Build history of the part. All positions in model axes, mm. A direction names the side the tool comes from. Round coordinates to 2 decimals unless told otherwise and drop trailing zeros. Order: outer loops, then holes, each group sorted by start corner. A loop starts at its lowest first (then second) coordinate and runs counter-clockwise, first axis right, second up. Notation, with made-up numbers: (37, 43) -> (70, 43) arc R21 cw to (70, 62) -> close; hole circle Ø10 at (-39.5, -21). An arc over 180 degrees is marked (long way). Use a Markdown table: item, result. Add a question column.
Item 1: Slice it at B-B, the plane z = -42. Give the cut face in (x, y), plus the area to 3 significant figures.
Item 2: 3-axis set-ups, long thin cutter, end or side, ignore diameter. For faces 1 (the face through (0, 2, -132)), 2 (the face through (20.5, 2, 2)), 3 (the face through (83, 2, 0)), 4 (the face through (45, 2, 4.5)), 5 (the face through (34, 0, -57)): which of +Z, -Z, +X, -X, +Y, -Y reach the whole face in a straight line?
Item 3: Slice it at A-A, the plane y = 1.6. Give the cut face in (x, z).
Item 4: Probe L1, parallel to Z at x = 23, y = 3.8; L2, parallel to Z at x = 42, y = 1.8; L3, parallel to X at y = 0.45, z = -63.5. List the from-to ranges inside material, lowest first.
Item 5: Pin check, flat tips, straight feed: pin 1 (2 mm diameter, centred on x = 19, y = 3, fed in from +Z); pin 2 (1.3 mm diameter, centred on y = 2, z = 2.5, fed in from -X); pin 3 (10 mm diameter, centred on x = 19, z = -128.5, fed in from +Y). Stop position of each tip, or through.
Item 6: Slice it at C-C, the plane x = 69. Give the cut face in (y, z).
from build123d import *

# Parameters (mm, degrees)
SKETCH1_W           = 4.5
SKETCH1_H           = 75
SKETCH1_W_2         = 50
SKETCH1_H_2         = 4.5
BOSS_EXTRUDE1_DEPTH = 4.5


with BuildPart() as part:
    # Sketch1 → Boss-Extrude1 (new body)
    with BuildSketch(Plane(origin=(0, 0, 0), x_dir=(1, 0, 0), z_dir=(0, 1, 0))):
        with Locations((-2.25, 75)):
            Rectangle(SKETCH1_W, SKETCH1_H)
        Polygon((0, 37.5), (0, 0), (20.5, 0), (20.5, 4.5), (70.5, 4.5), (70.5, 0), (95.5, 0), (0, 150), (0, 112.5), (4.5, 112.5), (4.5, 37.5), align=None)
        with Locations((45.5, -2.25)):
            Rectangle(SKETCH1_W_2, SKETCH1_H_2)
        with Locations((45.5, 2.25)):
            Rectangle(SKETCH1_W_2, SKETCH1_H_2)
        with Locations((2.25, 75)):
            Rectangle(SKETCH1_W, SKETCH1_H)
    extrude(amount=BOSS_EXTRUDE1_DEPTH)


solid = part.part
Check sheet entries:
| question | item | result |
|---|---|---|
| 1 | outline | (-4.5, 0) -> (68.76, 0) -> (68.76, 4.5) -> (-4.5, 4.5) -> close |
| 1 | area | 330 mm2 |
| 2 | face 1 | -Z, -X, +Y, -Y |
| 2 | face 2 | +Z, -X, +Y, -Y |
| 2 | face 3 | +Z, +X, +Y, -Y |
| 2 | face 4 | +Z, +X, -X, +Y, -Y |
| 2 | face 5 | +Z, -Z, +X, -X, -Y |
| 3 | outline | (-4.5, -112.5) -> (0, -112.5) -> (0, -150) -> (95.5, 0) -> (70.5, 0) -> (70.5, 4.5) -> (20.5, 4.5) -> (20.5, 0) -> (0, 0) -> (0, -37.5) -> (-4.5, -37.5) -> close |
| 4 | L1 | -113.87 to 4.5 |
| 4 | L2 | -84.03 to 4.5 |
| 4 | L3 | -4.5 to 55.07 |
| 5 | pin 1 | z = 0 |
| 5 | pin 2 | x = 20.5 |
| 5 | pin 3 | y = 4.5 |
| 6 | outline | (0, -41.62) -> (4.5, -41.62) -> (4.5, 4.5) -> (0, 4.5) -> close |
